from build123d import *

# Parameters (mm, degrees)
F0_W     = 152.4
F0_H     = 45.182696
F1_DEPTH = 63.5
F2_SIZE  = 25.4


with BuildPart() as f1:
    # F0 (on Right) → F1 (new body)
    with BuildSketch(Plane.YZ):
        Rectangle(F0_W, F0_H)
    extrude(amount=-F1_DEPTH)

    # F2
    f2_edges = [f1.edges().sort_by_distance(p)[0] for p in [
        (-31.75, -76.2, 22.591348),
    ]]
    chamfer(f2_edges, length=F2_SIZE)


solid = f1.part
Source: CAD feature listing. Evaluate the final solid. Frame: model axes, mm. Coordinates: 2 decimals unless noted, no trailing zeros. Loops run counter-clockwise (first coordinate to the right, second up) from the corner with the lowest first, then second, coordinate; pieces in that order, holes last. Notation, with made-up numbers: (-22, -4.75) - (-2, -4.75) arc R26 cw to (-2, 30.25) - close; hole circle Ø4 at (-8, 20.25). An arc over 180 degrees is marked (long way). Return JSON: item names as keys, results as strings.
Q1. Section C-C, the plane z = 18. Return loops of the section in (x, y), plus the area to 3 significant figures.
Results:
{"outline": "(-63.5, -55.39) - (0, -55.39) - (0, 76.2) - (-63.5, 76.2) - close", "area": "8,360 mm2"}
Q2. Mould query, pull axis Y, two halves, no side actions, for faces 1 (the flat face through (-31, -76.2, -13)), 2 (the flat face through (-31, 76.2, 0)), 3 (the flat face through (-63.5, -1, 0)). Classes: released by +Y, released by -Y, zero draft, split by the parting line, or undercut.
Results:
{"face 1": "released by -Y", "face 2": "released by +Y", "face 3": "zero draft"}
Q3. Section B-B, the plane z = 9. Return loops of the section in (x, y), plus the area to 3 significant figures.
Results:
{"outline": "(-63.5, -64.39) - (0, -64.39) - (0, 76.2) - (-63.5, 76.2) - close", "area": "8,930 mm2"}
Q4. Section A-A, the plane x = -14. Return loops of the section in (y, z), plus the area to 3 significant figures.
Results:
{"outline": "(-76.2, -22.59) - (76.2, -22.59) - (76.2, 22.59) - (-50.8, 22.59) - (-76.2, -2.81) - close", "area": "6,560 mm2"}
Q5. Contact query for flat-ended pins moving along their axis: P1, Ø4, axis at x = -13, z = 6.5, coming from the -Y side; P2, Ø12, axis at x = -44, z = 9.5, coming from the -Y side. Output: stop coordinate, or through.
Results:
{"P1": "y = -68.89", "P2": "y = -69.89"}
Q6. Material intervals for line 1 along Z through (x, y) = (-51.5, -63); line 2 along Y through (x, z) = (-51.5, 2.5); line 3 along Y through (x, z) = (-22, 8), sorted ascending.
Results:
{"line 1": "-22.59 to 10.39", "line 2": "-70.89 to 76.2", "line 3": "-65.39 to 76.2"}
